Can you work these out from the drawing? Everything is in mm from the part's minimum corner. Round coordinates to 2 decimals unless told otherwise and drop trailing zeros. Write each loop counter-clockwise with the first axis right and the second up, starting at its lowest first coordinate (ties: lowest second). Pieces come first, ordered by that corner, then holes. Notation, with made-up numbers: (58.25, 72) -> (78.25, 72) arc R22 ccw to (78.25, 99) -> close; hole circle Ø7 at (29.5, -32). An arc over 180 degrees is marked (long way). Write item = value, one per line. Start each with the question number.
1) Imagine slicing it at C-C, the plane x = 33. Please give me the cut outline in (y, z) (1 decimal), then the cut area to 3 significant figures.
2) Imagine slicing it at A-A, the plane x = 42.5. Please give me the cut outline in (y, z) (1 decimal).
3) If I drill on line 1 (X direction, y = 39.5, z = 1.6) (1 decimal); line 2 (Y direction, x = 31, z = 1.8) (1 decimal); line 3 (Y direction, x = 42, z = 2.5), over which ranges is the centre line in solid material (lowest first)?
4) I'm going to push flat-ended pins straight in: pin 1 (1.9 mm diameter, centred on x = 26.94, y = 38.1, fed in from +Z); pin 2 (6 mm diameter, centred on x = 34.5, y = 55, fed in from -Z); pin 3 (1 mm diameter, centred on y = 67.5, z = 2, fed in from +X). Where does each tip first touch, or does it pass through?
5) Imagine slicing it at D-D, the plane y = 26.5. Please give me the cut outline in (x, z) (1 decimal).
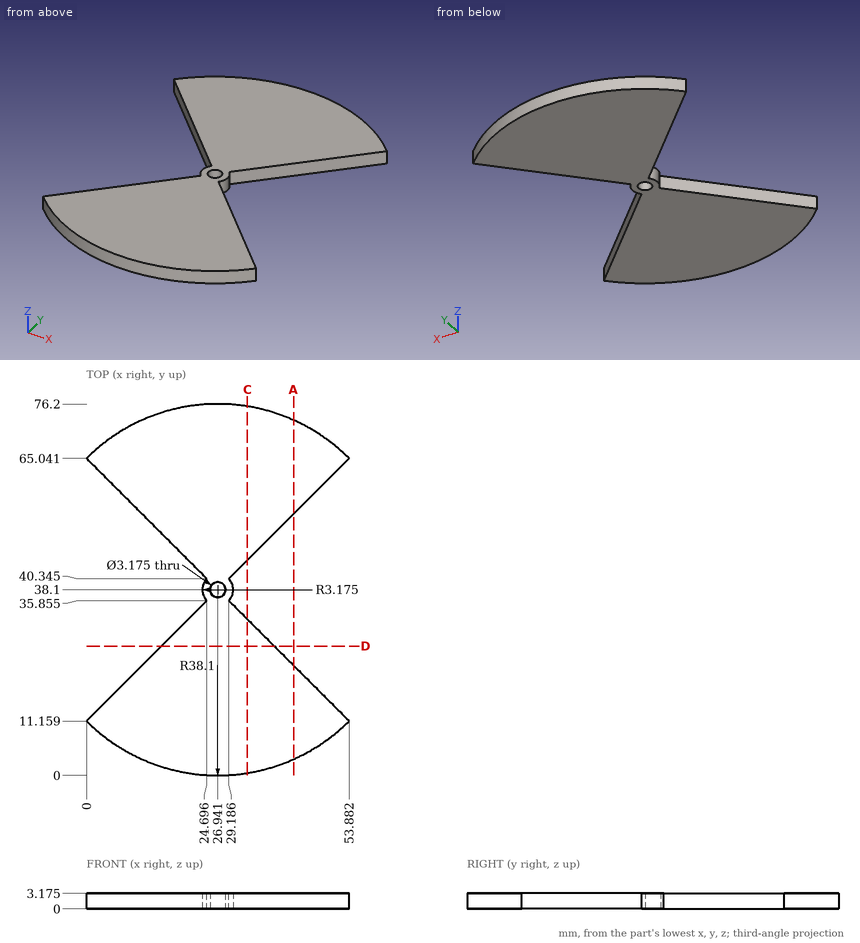
Reported:
q1.outline = (0.5, 0) -> (32, 0) -> (32, 3.2) -> (0.5, 3.2) -> close; (44.2, 0) -> (75.7, 0) -> (75.7, 3.2) -> (44.2, 3.2) -> close
q1.area = 200 mm²
q2.outline = (3.3, 0) -> (22.5, 0) -> (22.5, 3.2) -> (3.3, 3.2) -> close; (53.7, 0) -> (72.9, 0) -> (72.9, 3.2) -> (53.7, 3.2) -> close
q3.line_1 = 24.1 to 26.2, 27.7 to 29.8
q3.line_2 = 0.2 to 34, 42.2 to 76
q3.line_3 = 3.1 to 23.04, 53.16 to 73.1
q4.pin_1 = through
q4.pin_2 = 0
q4.pin_3 = 51.77
q5.outline = (15.3, 0) -> (38.5, 0) -> (38.5, 3.2) -> (15.3, 3.2) -> close
